For this review, take the finished solid that the model builds, in its own axes (mm). A direction names the side the tool comes from. Coordinates: 2 decimals unless noted, no trailing zeros. Write each loop counter-clockwise with the first axis right and the second up, starting at its lowest first coordinate (ties: lowest second). Pieces come first, ordered by that corner, then holes. Notation, with made-up numbers: M -12,33 L 34,33 A21 ccw 34,55 Z; hole C 78.5,13 d6. An arc over 180 degrees is marked long. Return JSON: item names as keys, results as strings.
```python
from build123d import *

# Parameters (mm, degrees)
CROQUIS1_W              = 101
CROQUIS1_H              = 70
CROQUIS1_W_2            = 89
CROQUIS1_H_2            = 58
CROQUIS1_H_3            = 6
SALIENTE_EXTRUIR1_DEPTH = 3
SALIENTE_EXTRUIR2_DEPTH = 10
CROQUIS3_W              = 5
CROQUIS3_H              = 6
SALIENTE_EXTRUIR3_DEPTH = 10
REDONDEO1_R             = 10
REDONDEO2_R             = 3
CROQUIS5_W              = 40
CROQUIS5_H              = 6
SALIENTE_EXTRUIR4_DEPTH = 15
CROQUIS6_R              = 2.45
SALIENTE_EXTRUIR5_DEPTH = 8
CROQUIS7_W              = 22
CROQUIS7_H              = 6
SALIENTE_EXTRUIR6_DEPTH = 10
CROQUIS8_R              = 5
SALIENTE_EXTRUIR7_DEPTH = 5
CROQUIS9_W              = 22
CROQUIS9_H              = 19.446808743
CORTAR_EXTRUIR1_DEPTH   = 119.004237212
CROQUIS10_W             = 28.262492251
CROQUIS10_H             = 3.390066726
CORTAR_EXTRUIR2_DEPTH   = 8


with BuildPart() as part:
    # Croquis1 → Saliente-Extruir1 (new body)
    # profile 1 of 3: a face of its own
    with BuildSketch(Plane.XY):
        with Locations((47.5, 32)):
            Rectangle(CROQUIS1_W, CROQUIS1_H)
        with Locations((47.5, 32)):
            Rectangle(CROQUIS1_W_2, CROQUIS1_H_2, mode=Mode.SUBTRACT)
    # profile 2 of 3: a face of its own
    with BuildSketch(Plane.XY):
        with Locations((47.5, 48)):
            Rectangle(CROQUIS1_W_2, CROQUIS1_H_3)
    # profile 3 of 3: a face of its own
    with BuildSketch(Plane.XY):
        with Locations((47.5, 25.4)):
            Rectangle(CROQUIS1_W_2, CROQUIS1_H_3)
    extrude(amount=SALIENTE_EXTRUIR1_DEPTH)

    # Croquis2 → Saliente-Extruir2 (add)
    with BuildSketch(Plane.XY.offset(3)):
        Polygon((85, 67), (98, 67), (98, 54), (95, 54), (95, 64), (85, 64), align=None)
        Polygon((10, 64), (10, 67), (-3, 67), (-3, 54), (0, 54), (0, 64), align=None)
        Polygon((10, -3), (-3, -3), (-3, 10), (0, 10), (0, 0), (10, 0), align=None)
        Polygon((85, 0), (85, -3), (98, -3), (98, 10), (95, 10), (95, 0), align=None)
    extrude(amount=SALIENTE_EXTRUIR2_DEPTH)

    # Croquis3 → Saliente-Extruir3 (add)
    with BuildSketch(Plane.XY.offset(3)):
        with Locations((56, 48)):
            Rectangle(CROQUIS3_W, CROQUIS3_H)
        with Locations((39, 48)):
            Rectangle(CROQUIS3_W, CROQUIS3_H)
    extrude(amount=SALIENTE_EXTRUIR3_DEPTH)

    # Redondeo1
    redondeo1_edges = [part.edges().sort_by_distance(p)[0] for p in [
        (36.5, 48, 3),
        (58.5, 48, 3),
    ]]
    fillet(redondeo1_edges, radius=REDONDEO1_R - 0.0001)  # a hair under: the kernel refuses the full size

    # Redondeo2
    redondeo2_edges = [part.edges().sort_by_distance(p)[0] for p in [
        (85, -1.5, 3),
        (96.5, 10, 3),
        (85, 65.5, 3),
        (96.5, 54, 3),
        (10, 65.5, 3),
        (-1.5, 54, 3),
        (10, -1.5, 3),
        (-1.5, 10, 3),
    ]]
    fillet(redondeo2_edges, radius=REDONDEO2_R)

    # Croquis5 → Saliente-Extruir4 (add)
    with BuildSketch(Plane(origin=(0, 0, 0), x_dir=(-1, 0, 0), z_dir=(0, 0, -1))):
        with Locations((-47.5, 25.4)):
            Rectangle(CROQUIS5_W, CROQUIS5_H)
    extrude(amount=SALIENTE_EXTRUIR4_DEPTH)

    # Croquis6 → Saliente-Extruir5 (add)
    with BuildSketch(Plane(origin=(0, 28.4, 0), x_dir=(1, 0, 0), z_dir=(0, 1, 0))):
        with Locations(Location((35.5, 7, 0), (0, 0, 270))):
            Circle(CROQUIS6_R)
        with Locations(Location((59.5, 7, 0), (0, 0, 270))):
            Circle(CROQUIS6_R)
    extrude(amount=SALIENTE_EXTRUIR5_DEPTH)

    # Croquis7 → Saliente-Extruir6 (add, through all)
    with BuildSketch(Plane.XY.offset(3)):
        with Locations((47.5, 0)):
            Rectangle(CROQUIS7_W, CROQUIS7_H)
        with Locations((47.5, 64)):
            Rectangle(CROQUIS7_W, CROQUIS7_H)
    extrude(amount=SALIENTE_EXTRUIR6_DEPTH)

    # Croquis8 → Saliente-Extruir7 (add)
    with BuildSketch(Plane.XZ.offset(3)):
        with Locations(Location((47.5, 9, 0), (0, 0, 126.869897646))):
            Circle(CROQUIS8_R)
    saliente_extruir7 = extrude(amount=SALIENTE_EXTRUIR7_DEPTH)

    # Croquis9 → Cortar-Extruir1 (cut, through all)
    with BuildSketch(Plane(origin=(0, 3, 0), x_dir=(1, 0, 0), z_dir=(0, 1, 0))):
        with Locations((47.5, -22.723404372)):
            Rectangle(CROQUIS9_W, CROQUIS9_H)
    cortar_extruir1 = extrude(amount=-CORTAR_EXTRUIR1_DEPTH, mode=Mode.SUBTRACT)

    # Simetría1: Saliente-Extruir7, Cortar-Extruir1 across plane
    add(saliente_extruir7.mirror(Plane.ZX.offset(31)))
    add(cortar_extruir1.mirror(Plane.ZX.offset(31)), mode=Mode.SUBTRACT)

    # Croquis10 → Cortar-Extruir2 (cut)
    with BuildSketch(Plane(origin=(0, 36.4, 0), x_dir=(1, 0, 0), z_dir=(0, 1, 0))):
        with Locations((47.340282602, 3.804966637)):
            Rectangle(CROQUIS10_W, CROQUIS10_H)
    extrude(amount=-CORTAR_EXTRUIR2_DEPTH, mode=Mode.SUBTRACT)


solid = part.part
```
1. We need section B-B (x = 47.5). State the section outline as (y, z) points.
Checks:
{"outline": "M -8,4 L -3,4 L -3,0 L 3,0 L 3,13 L -8,13 Z; M 22.4,-15 L 28.4,-15 L 28.4,3 L 22.4,3 Z; M 45,0 L 51,0 L 51,3 L 45,3 Z; M 61,0 L 67,0 L 67,4 L 70,4 L 70,13 L 61,13 Z"}
2. We need section C-C (x = 88). State the section outline as (y, z) points.
Checks:
{"outline": "M -3,0 L 3,0 L 3,3 L 0,3 L 0,13 L -3,13 Z; M 22.4,0 L 28.4,0 L 28.4,3 L 22.4,3 Z; M 45,0 L 51,0 L 51,3 L 45,3 Z; M 61,0 L 67,0 L 67,13 L 64,13 L 64,3 L 61,3 Z"}
3. We need section A-A (y = 58). State the section outline as (x, z) points.
Checks:
{"outline": "M -3,0 L 3,0 L 3,3 L 0,3 L 0,13 L -3,13 Z; M 92,0 L 98,0 L 98,13 L 95,13 L 95,3 L 92,3 Z"}
4. We need section D-D (z = 8.5). Give the number of separate pieces and of enclosed holes in the cut face, plus the area to 3 significant figures.
Checks:
{"separate pieces": "8", "enclosed holes": "0", "area": "692 mm2"}
5. Draft analysis for pull direction Y (two halves, no side actions). For faces 1 (the face through (92, 56, 1)), 2 (the face through (47, -8, 9)), 3 (the face through (10.9, 65.52, 3.86)), state which applies: +Y half, -Y half, draft (parallel to the pull), parting line (faces both ways), or undercut.
Checks:
{"face 1": "undercut", "face 2": "-Y half", "face 3": "draft"}
6. Clearance check with flat-ended pins moving along their axes: pin 1 Ø5.5 at (x, z) = (34.5, -6.5) entering from +Y; pin 2 Ø1.5 at (x, z) = (96, 8) entering from -Y; pin 3 Ø5 at (y, z) = (49, 7) entering from +X. State where each tip first meets the part, or that it passes through.
Checks:
{"pin 1": "y = 36.4", "pin 2": "y = -3", "pin 3": "x = 63.23"}
7. For faces 4 (the face through (35, 32, -5.5)), 5 (the face through (-2, 54, 9)), 6 (the face through (95, 59, 8)), list the 3-axis set-ups (+Z, -Z, +X, -X, +Y, -Y) from which the entire face can be reached by the end or side of a thin tool; tool diameter is ignored.
Checks:
{"face 4": "+Z, +X, -X, +Y", "face 5": "+Z, +X, -X", "face 6": "+Z"}
8. Wall thickness on L1, parallel to Y at x = 54, z = 3.5; L2, parallel to Y at x = 69.5, z = 0.75; L3, parallel to X at y = 40, z = 1.5: over which ranges is each line inside the solid? List them lowest first. Write a range as from..to.
Checks:
{"L1": "-3..3, 45..51, 61..67", "L2": "-3..3, 22.4..28.4, 45..51, 61..67", "L3": "-3..3, 92..98"}
